Verification items for the finished model (mm, model axes). A direction names the side the tool comes from. Round coordinates to 2 decimals unless told otherwise and drop trailing zeros. Write each loop counter-clockwise with the first axis right and the second up, starting at its lowest first coordinate (ties: lowest second). Pieces come first, ordered by that corner, then holes. Notation, with made-up numbers: (70.5, 36) -> (106.5, 36) arc R18 ccw to (106.5, 61) -> close; hole circle Ø4 at (13, -19). An arc over 180 degrees is marked (long way). Use CSV: the item, a comma, the result in double quotes.
Autodesk Inventor part; units mm, degrees
ref_plane "YZ Plane" through (0, 0, 0) normal (1, 0, 0) x (0, 1, 0)
ref_plane "XZ Plane" through (0, 0, 0) normal (0, 1, 0) x (-1, 0, 0)
ref_plane "XY Plane" through (0, 0, 0) normal (0, 0, 1) x (1, 0, 0)
sketch "Sketch1" plane through (0, 0, 0) normal (0, 0, 1) x (1, 0, 0)
  circle A0 centre (-5, -11) radius 3
  circle A1 centre (5, 11) radius 3
  point P0 (0, 0)
  dimension "d0" = 10
  dimension "d1" = 22
  dimension "d2" = 5
  dimension "d3" = 11
  dimension "d4" = 6
  dimension "d5" = 6
extrude "Extrusion1" add sketch "Sketch1" along normal blind 8
sketch "Sketch2" plane through (5, 11, 8) normal (0, 0, 1) x (1, 0, 0)
  circle A0 centre (0, 0) radius 3
  circle A1 centre (-10, -22) radius 3
  line L0 (-10, -22) -> (-8.5, -18) construction
  line L1 (-9.0637, -22.3511) -> (-7.5637, -18.3511)
  line L2 (-9.4363, -17.6489) -> (-10.9363, -21.6489)
  arc A2 (-10.9363, -21.6489) -> (-9.0637, -22.3511) centre (-10, -22) ccw
  arc A3 (-7.5637, -18.3511) -> (-9.4363, -17.6489) centre (-8.5, -18) ccw
  circle A4 centre (-8.5, 0) radius 1
  point P0 (-5, -11)
  point P1 (-10, -19)
  point P2 (-9.25, -20)
  dimension "d8" = 0
  dimension "d9" = 1.5
  dimension "d10" = 3
  dimension "d11" = 0
  dimension "d12" = 1.5
  dimension "d13" = 4
  dimension "d14" = 2
  dimension "d15" = 2
extrude "Extrusion2" add sketch "Sketch2" against normal blind 8 contours L1 A2 L2 A1 | A1 L2 A3 L1 | A4 picked at (-9.757, -21.03)
sketch "Sketch3" plane through (-3.5, 11, 8) normal (0, 0, 1) x (1, 0, 0)
  circle A0 centre (0, 0) radius 1
  circle A1 centre (8.5, 0) radius 3
  line L0 (0, 0) -> (8.5, 0) construction
  line L1 (0, -1) -> (8.5, -1)
  line L2 (8.5, 1) -> (0, 1)
  arc A2 (0, 1) -> (0, -1) centre (0, 0) ccw
  arc A3 (8.5, -1) -> (8.5, 1) centre (8.5, 0) ccw
  arc A4 (0.9363, -18.3511) -> (-0.9363, -17.6489) centre (0, -18) ccw
  line L3 (0, 0) -> (0, -18) construction
  line L4 (-1, 0) -> (-1, -18)
  line L5 (1, -18) -> (1, 0)
  arc A5 (1, 0) -> (-1, 0) centre (0, 0) ccw
  arc A6 (-1, -18) -> (1, -18) centre (0, -18) ccw
  point P0 (3.5, -11)
  point P1 (4.25, 0)
  point P2 (0, -9)
  point P3 (1, -1)
  point P4 (-1, 0)
extrude "Extrusion3" add sketch "Sketch3" against normal blind 8 contours A0 | L5 L1 A0 | A0 L2 A1 L1 L5 | L1 L5 A4 A6 L4 A0 | L2 A3 L1 A1 picked at (7.5064, 0.113)
fillet "Fillet1" radius 2 1 edges at (-2.5, 10, 4)
fillet "Fillet2" radius 2 4 edges at (2.1716, 10, 4) (-4.9432, -8.0005, 4) (-3.0705, -8.7028, 4) (2.1716, 12, 4)
sketch "Sketch4" plane through (0, 0, 0) normal (0, 0, -1) x (-1, 0, 0)
  arc A0 (-2.6, 12.8) -> (-2.6, 9.2) centre (-5, 11) ccw
  arc A1 (2.4719, -9.3848) -> (5.8427, -8.1208) centre (5, -11) ccw
  point P0 (0, 0)
hole "Hole1" at (5, 11, 0) at (-5, -11, 0) direction (0, 0, 1) diameter 2 depth 5 tip angle 118
sketch "Sketch5" plane through (0, 0, 8) normal (0, 0, 1) x (1, 0, 0)
  circle A0 centre (5, 11) radius 1
  circle A1 centre (-5, -11) radius 1
  point P0 (0, 0)
hole "Hole2" at (5, 11, 8) at (-5, -11, 8) direction (0, 0, -1) diameter 2 depth 5 tip angle 118
properties part number "back"
Q1. Section check C-C (y = -3.75). Record the cut outline in (x, z), plus the area to 3 significant figures.
Filled in:
outline,"(-4.5, 0) -> (-2.5, 0) -> (-2.5, 8) -> (-4.5, 8) -> close"
area,"16.0 mm²"
Q2. Material ranges on L1, parallel to Y at x = 5, z = 2.1; L2, parallel to X at y = 11, z = 6.45; L3, parallel to X at y = -11, z = 6.9, recorded low to high.
Filled in:
L1,"8 to 10, 12 to 14"
L2,"-4.5 to 4, 6 to 8"
L3,"-8 to -6, -4 to -2"
Q3. Mould release check, pull along Y, two halves, no side actions. Record for faces 6 (the cylindrical face through (8, 11, 4)), 7 (the flat face through (-2.5, 0, 4)), 8 (the cylindrical face through (-5.034, -7.658, 3.944)), 9 (the flat face through (-3, 1, 0)): released by +Y, released by -Y, zero draft, split by the parting line, or undercut.
Filled in:
face 6,"split by the parting line"
face 7,"undercut"
face 8,"released by +Y"
face 9,"zero draft"
Q4. Access from +Z, -Z, +X, -X, +Y, -Y to the whole of each face (thin tool, end or side, straight path). Record for faces 1 (the flat face through (-3, 1, 8)), 2 (the flat face through (-4.5, 2, 4)), 3 (the cylindrical face through (-2.774, -8.53, 3.944)), 4 (the cylindrical face through (-1.93, 9.4, 3.94)), 5 (the cylindrical face through (1.883, 9.795, 3.944)).
Filled in:
face 1,"+Z, +X, -X, +Y, -Y"
face 2,"+Z, -Z, -X, +Y"
face 3,"+Z, -Z, +X"
face 4,"+Z, -Z"
face 5,"+Z, -Z, -Y"
Q5. Section check A-A (y = -11). Record the cut outline in (x, z).
Filled in:
outline,"(-8, 0) -> (-6, 0) -> (-6, 8) -> (-8, 8) -> close; (-4, 0) -> (-2, 0) -> (-2, 8) -> (-4, 8) -> close"
Q6. Section check D-D (y = 9.5). Record the cut outline in (x, z).
Filled in:
outline,"(-4.5, 0) -> (-1.82, 0) -> (-1.82, 8) -> (-4.5, 8) -> close; (2.32, 0) -> (7.6, 0) -> (7.6, 8) -> (2.32, 8) -> close"
Q7. Section check B-B (z = 7). Record the cut outline in (x, y).
Filled in:
outline,"(-5.84, -8.12) arc R3 ccw (long way) to (-2.47, -9.38) arc R2 cw to (-2.66, -7.61) -> (-2.56, -7.35) arc R1 ccw to (-2.5, -7) -> (-2.5, 8) arc R2 cw to (-0.5, 10) -> (1, 10) arc R2 cw to (2.6, 9.2) arc R3 ccw (long way) to (2.6, 12.8) arc R2 cw to (1, 12) -> (-3.5, 12) arc R1 ccw to (-4.5, 11) -> (-4.5, -6.82) -> (-4.53, -6.9) arc R2 cw to start; hole circle Ø2 at (-5, -11); hole circle Ø2 at (5, 11)"
Q8. Go/stop test with flat-tipped pins: P1, Ø8, axis at x = -0.5, y = -8.5, coming from the -Z side; P2, Ø2, axis at y = 6, z = 2.5, coming from the +X side; P3, Ø4, axis at y = 7, z = 6, coming from the -X side; P4, Ø8, axis at x = 4, y = 0, coming from the -Z side. Record where each tip stops, or that it passes through.
Filled in:
P1,"z = 0"
P2,"x = -2.5"
P3,"x = -4.5"
P4,"through"
